Here's how the part is built. I have some questions about the finished solid (model axes, mm). A direction names the side the tool comes from. Round coordinates to 2 decimals unless told otherwise and drop trailing zeros. Loops run counter-clockwise (first coordinate to the right, second up) from the corner with the lowest first, then second, coordinate; pieces in that order, holes last. Notation, with made-up numbers: M 79.25,-21 L 84.25,-21 A29 ccw 84.25,6 Z; hole C 48.25,8 d8. An arc over 180 degrees is marked long. Use a Markdown table: item, result.
Autodesk Inventor part; units mm, degrees
ref_plane "YZ Plane" through (0, 0, 0) normal (1, 0, 0) x (0, 1, 0)
ref_plane "XZ Plane" through (0, 0, 0) normal (0, 1, 0) x (-1, 0, 0)
ref_plane "XY Plane" through (0, 0, 0) normal (0, 0, 1) x (1, 0, 0)
sketch "Sketch1" plane through (0, 0, 0) normal (0, 0, 1) x (1, 0, 0)
  circle A0 centre (0, 0) radius 190
  circle A1 centre (0, 0) radius 301
  circle A2 centre (0, 0) radius 265 construction
  point P0 (0, 265)
  dimension "d17" = 530
  dimension "d41" = 602
  dimension "d42" = 380
extrude "Extrusion1" add sketch "Sketch1" along normal blind 15
sketch "Sketch2" plane through (0, 0, 15) normal (0, 0, 1) x (1, 0, 0)
  circle A0 centre (0, 0) radius 301 construction
  circle A1 centre (0, 0) radius 190 construction
  line L0 (0, 286) -> (0, 244) construction
  line L1 (0, 190) -> (0, 0) construction
  circle A2 centre (0, 0) radius 244
  circle A3 centre (0, 0) radius 286
  circle A4 centre (0, 0) radius 265 construction
  point P0 (0, 265)
  dimension "d19" = 530
  dimension "d4" = 42
extrude "Extrusion2" cut sketch "Sketch2" against normal blind 3.5
sketch "Sketch3" plane through (0, 0, 0) normal (0, 0, 1) x (1, 0, 0)
  circle A0 centre (0, 0) radius 190 construction
  circle A1 centre (0, 0) radius 301 construction
  circle A2 centre (0, 0) radius 244
  circle A3 centre (0, 0) radius 286
  circle A4 centre (0, 0) radius 301
  line L0 (0, 0) -> (0, -301) construction
  line L1 (0, 0) -> (58.7222, -295.2164) construction
  line L2 (47.602, -239.3116) -> (55.7958, -280.5046) construction
  circle A5 centre (51.6989, -259.9081) radius 7
  dimension "d20" = 11.25
  dimension "d21" = 14
extrude "Extrusion3" cut sketch "Sketch3" along normal through all contours A5
pattern_circular "Circular Pattern2" count 16 over 360 about axis through (0, 0, 0) along (0, 0, -1) of "Extrusion3"
sketch "Sketch5" plane through (0, 0, 0) normal (0, 0, -1) x (-1, 0, 0)
  circle A0 centre (0, 0) radius 301
  circle A1 centre (0, 0) radius 190
  line L0 (0, 0) -> (0, 190) construction
  arc A2 (2.9999, 189.9763) -> (-2.9999, 189.9763) centre (0, 190) ccw
  dimension "d40" = 6
extrude "Extrusion4" cut sketch "Sketch5" against normal through all contours A1 A2
mirror "Mirror1" about plane through (0, 0, 0) normal (0, 1, 0) of "Extrusion4"
equation "\"d17\" = Шпил_пласт_КОРМА_диам_центров"
equation "\"d19\" = Шпил_пласт_КОРМА_диам_центров"
equation "\"BendReliefDepth\" = 0.5 * Thickness"
properties part number "ДМФ 025 кольцо прижимное корма наружное"
Q1. Will these pins go through, and if not, where does the flat tip stop? P1, Ø11, axis at x = 259.91, y = 51.7, coming from the -Z side; P2, Ø1.5, axis at x = -130.5, z = 9, coming from the +Y side; P3, Ø2, axis at x = 225, z = 13, coming from the +Y side; P4, Ø4, axis at x = -61, z = 5.5, coming from the +Y side.
Return value:
| item | result |
|---|---|
| P1 | passes through |
| P2 | stops at y = 271.6 |
| P3 | stops at y = 201.06 |
| P4 | stops at y = 295.16 |
Q2. Imagine slicing it at C-C, the plane z = 8.5. Give the number of separate pieces and of enclosed holes in the cut face, then the cut area to 3 significant figures.
Return value:
| item | result |
|---|---|
| separate pieces | 1 |
| enclosed holes | 17 |
| area | 169,000 mm^2 |
Q3. We'd pull the mould along Y, two halves only. Please class faces 1 (the cylindrical face through (-221.85, -203.43, 7.4)), 2 (the flat face through (-4, -196, 0)), 3 (the cylindrical face through (-193.63, -148.47, 13.27)): pulls with the +Y half, pulls with the -Y half, needs draft (parallel to the pull), parting line crosses it, or undercut.
Return value:
| item | result |
|---|---|
| face 1 | parting line crosses it |
| face 2 | needs draft |
| face 3 | undercut |
Q4. For faces 4 (the cylindrical face through (-189.955, -4.136, 7.395)), 5 (the flat face through (211, 128, 11.5)), which set-ups out of +Z, -Z, +X, -X, +Y, -Y let a thin tool reach every point of the face, with its end or its side?
Return value:
| item | result |
|---|---|
| face 4 | +Z, -Z |
| face 5 | +Z |
Q5. Imagine slicing it at B-B, the plane x = 181. Please give me the cut outline in (y, z), then the cut area to 3 significant figures.
Return value:
| item | result |
|---|---|
| outline | M -240.5,0 L -57.78,0 L -57.78,15 L -163.63,15 L -163.63,11.5 L -221.44,11.5 L -221.44,15 L -240.5,15 Z; M 57.78,0 L 240.5,0 L 240.5,15 L 221.44,15 L 221.44,11.5 L 163.63,11.5 L 163.63,15 L 57.78,15 Z |
| area | 5,080 mm^2 |
Q6. Imagine slicing it at A-A, the plane y = 0. Please give me the cut outline in (x, z), then the cut area to 3 significant figures.
Return value:
| item | result |
|---|---|
| outline | M -301,0 L -190,0 L -190,15 L -244,15 L -244,11.5 L -286,11.5 L -286,15 L -301,15 Z; M 190,0 L 301,0 L 301,15 L 286,15 L 286,11.5 L 244,11.5 L 244,15 L 190,15 Z |
| area | 3,040 mm^2 |
Q7. I need wall thicknesses on line 1 (Y direction, x = 79, z = 13); line 2 (Y direction, x = 82, z = 12.25); line 3 (Y direction, x = -259, z = 9). Which ranges of each line are inside material? Lowest first, please. Write a range as from..to.
Return value:
| item | result |
|---|---|
| line 1 | y = -290.45..-274.87, -230.86..-172.8, 172.8..230.86, 274.87..290.45 |
| line 2 | y = -289.62..-273.99, -229.81..-171.39, 171.39..229.81, 273.99..289.62 |
| line 3 | y = -153.36..-58.64, -44.76..44.76, 58.64..153.36 |
